The listing builds one solid part. Answer for the finished solid, in the listing's coordinates (mm). Face numbers are marked on the shaded views. Coordinates: 2 decimals unless noted, no trailing zeros. Order: outer loops, then holes, each group sorted by start corner. A loop starts at its lowest first (then second) coordinate and runs counter-clockwise, first axis right, second up.
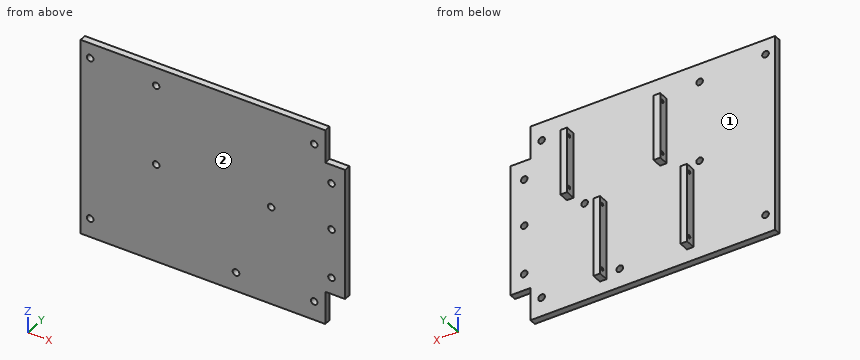
from build123d import *

# Parameters (mm, degrees)
SKETCH1_W               = 508
SKETCH1_H               = 381
BOSS_EXTRUDE1_DEPTH     = 12.7
SKETCH5_W               = 12.7
SKETCH5_H               = 127
BOSS_EXTRUDE2_DEPTH     = 19.05
SKETCH6_W               = 12.7
SKETCH6_H               = 127
BOSS_EXTRUDE3_DEPTH     = 19.05
SKETCH7_W               = 12.7
SKETCH7_H               = 152.4
BOSS_EXTRUDE6_DEPTH     = 19.05
CUT_EXTRUDE1_DEPTH      = 445.227773783
CUT_EXTRUDE1_DEPTH_BACK = 445.227773783
SKETCH8_R               = 3.175
CUT_EXTRUDE2_DEPTH      = 389.026049383
CUT_EXTRUDE2_DEPTH_BACK = 389.026049383
SKETCH9_R               = 3.175
SKETCH10_W              = 38.1
SKETCH10_H              = 63.5
CUT_EXTRUDE3_DEPTH      = 319.070986574
SKETCH11_W              = 38.1
SKETCH11_H              = 63.5
CUT_EXTRUDE4_DEPTH      = 319.070986574
CUT_EXTRUDE5_DEPTH      = 319.070986574
CUT_EXTRUDE5_DEPTH_BACK = 319.070986574
SKETCH13_R              = 6.35


with BuildPart() as part:
    # Sketch1 → Boss-Extrude1 (new body)
    with BuildSketch(Plane(origin=(0, 0, 0), x_dir=(1, 0, 0), z_dir=(0, 1, 0))):
        Rectangle(SKETCH1_W, SKETCH1_H)
    extrude(amount=BOSS_EXTRUDE1_DEPTH)

    # Sketch5 → Boss-Extrude2 (add)
    with BuildSketch(Plane(origin=(0, 12.7, 0), x_dir=(1, 0, 0), z_dir=(0, 1, 0))):
        with Locations((139.7, -82.55)):
            Rectangle(SKETCH5_W, SKETCH5_H)
    extrude(amount=BOSS_EXTRUDE2_DEPTH)

    # Sketch6 → Boss-Extrude3 (add)
    with BuildSketch(Plane(origin=(0, 12.7, 0), x_dir=(1, 0, 0), z_dir=(0, 1, 0))):
        with Locations((-39.37, -82.55)):
            Rectangle(SKETCH6_W, SKETCH6_H)
    extrude(amount=BOSS_EXTRUDE3_DEPTH)

    # Sketch7 → Boss-Extrude6 (add)
    with BuildSketch(Plane(origin=(0, 12.7, 0), x_dir=(1, 0, 0), z_dir=(0, 1, 0))):
        with Locations((76.2, 88.9)):
            Rectangle(SKETCH7_W, SKETCH7_H)
        with Locations((-90.932, 88.9)):
            Rectangle(SKETCH7_W, SKETCH7_H)
    extrude(amount=BOSS_EXTRUDE6_DEPTH)

    # Sketch8 → Cut-Extrude1 (cut, two sides: drawn at the far end of the back side and taken through both)
    with BuildSketch(Plane(origin=(146.05, 0, 0), x_dir=(0, 0, -1), z_dir=(1, 0, 0)).offset(-CUT_EXTRUDE1_DEPTH_BACK)):
        with Locations((-31.75, 25.4)):
            Circle(SKETCH8_R)
        with Locations((-133.35, 25.4)):
            Circle(SKETCH8_R)
    extrude(amount=CUT_EXTRUDE1_DEPTH + CUT_EXTRUDE1_DEPTH_BACK, mode=Mode.SUBTRACT)

    # Sketch9 → Cut-Extrude2 (cut, two sides: drawn at the far end of the back side and taken through both)
    with BuildSketch(Plane(origin=(82.55, 0, 0), x_dir=(0, 0, -1), z_dir=(1, 0, 0)).offset(-CUT_EXTRUDE2_DEPTH_BACK)):
        with Locations((25.4, 25.4)):
            Circle(SKETCH9_R)
        with Locations((152.4, 25.4)):
            Circle(SKETCH9_R)
    extrude(amount=CUT_EXTRUDE2_DEPTH + CUT_EXTRUDE2_DEPTH_BACK, mode=Mode.SUBTRACT)

    # Sketch10 → Cut-Extrude3 (cut, through all)
    with BuildSketch(Plane(origin=(0, 12.7, 0), x_dir=(1, 0, 0), z_dir=(0, 1, 0))):
        with Locations((234.95, -158.75)):
            Rectangle(SKETCH10_W, SKETCH10_H)
    extrude(amount=-CUT_EXTRUDE3_DEPTH, mode=Mode.SUBTRACT)

    # Sketch11 → Cut-Extrude4 (cut, through all)
    with BuildSketch(Plane(origin=(0, 12.7, 0), x_dir=(1, 0, 0), z_dir=(0, 1, 0))):
        with Locations((234.95, 158.75)):
            Rectangle(SKETCH11_W, SKETCH11_H)
    extrude(amount=-CUT_EXTRUDE4_DEPTH, mode=Mode.SUBTRACT)

    # Sketch13 → Cut-Extrude5 (cut, two sides: drawn at the far end of the back side and taken through both)
    with BuildSketch(Plane(origin=(0, 12.7, 0), x_dir=(1, 0, 0), z_dir=(0, 1, 0)).offset(-CUT_EXTRUDE5_DEPTH_BACK)):
        with Locations(Location((227.907081751, 0, 0), (0, 0, 270))):
            Circle(SKETCH13_R)
        with Locations(Location((111.925251719, 0, 0), (0, 0, 270))):
            Circle(SKETCH13_R)
        with Locations(Location((-108.969473195, 0, 0), (0, 0, 270))):
            Circle(SKETCH13_R)
        with Locations(Location((227.907081751, -90.673413336, 0), (0, 0, 270))):
            Circle(SKETCH13_R)
        with Locations(Location((227.907081751, 94.901161445, 0), (0, 0, 270))):
            Circle(SKETCH13_R)
        with Locations(Location((194.548146226, 154.151481102, 0), (0, 0, 270))):
            Circle(SKETCH13_R)
        with Locations(Location((194.548146226, -155.144429721, 0), (0, 0, 270))):
            Circle(SKETCH13_R)
        with Locations(Location((-235.634199607, -161.494429721, 0), (0, 0, 270))):
            Circle(SKETCH13_R)
        with Locations(Location((-235.634199607, 154.151481102, 0), (0, 0, 270))):
            Circle(SKETCH13_R)
        with Locations(Location((44.45, 154.151481102, 0), (0, 0, 270))):
            Circle(SKETCH13_R)
        with Locations(Location((-108.969473196, -155.144429721, 0), (0, 0, 270))):
            Circle(SKETCH13_R)
    extrude(amount=CUT_EXTRUDE5_DEPTH + CUT_EXTRUDE5_DEPTH_BACK, mode=Mode.SUBTRACT)


solid = part.part
1) Section B-B (z = 57) is taken. Give the vertices of the cut face in (x, y), then the cut area to 3 significant figures.
2) Section A-A (x = 44.45) is taken. Give the vertices of the cut face in (y, z).
3) Consider L1, parallel to Z at x = -91.75, y = 25.4 (3 decimals); L2, parallel to Z at x = 194.5, y = 9; L3, parallel to X at y = 26.5, z = -73. Determine where each line is inside the solid, lowest interval first.
4) Section D-D (y = 7.5) is taken. Give the number of separate pieces and of enclosed holes in the cut face, then the cut area to 3 significant figures.
5) Determine the mould class of the marked faces 1 and 2 for opening direction X: released by +X, released by -X, zero draft, split by the parting line, or undercut.
6) Each of these flat-tipped pins is pushed along its axis until it touches: P1, Ø20.5, axis at x = 111.93, z = 0, coming from the +Y side; P2, Ø10, axis at y = 25.4, z = 31.75, coming from the -X side; P3, Ø2, axis at x = -85.5, y = 14.5, coming from the -Z side. Where does it stop, or does it pass through?
7) Section C-C (z = 0) is taken. Give the vertices of the cut face in (x, y).
Filled sheet:
1. outline: (-254, 0) - (254, 0) - (254, 12.7) - (146.05, 12.7) - (146.05, 31.75) - (133.35, 31.75) - (133.35, 12.7) - (-33.02, 12.7) - (-33.02, 31.75) - (-45.72, 31.75) - (-45.72, 12.7) - (-254, 12.7) - close
1. area: 6,940 mm2
2. outline: (0, -190.5) - (12.7, -190.5) - (12.7, -160.5) - (0, -160.5) - close; (0, -147.8) - (12.7, -147.8) - (12.7, 190.5) - (0, 190.5) - close
3. L1: z = -165.1 to -155.575, -149.225 to -28.575, -22.225 to -12.7
3. L2: z = -190.5 to -160.5, -147.8 to 148.79, 161.49 to 190.5
3. L3: x = -97.28 to -84.58, 69.85 to 82.55
4. separate pieces: 1
4. enclosed holes: 11
4. area: 187,000 mm2
5. face 1: undercut
5. face 2: zero draft
6. P1: stops at y = 12.7
6. P2: stops at x = -45.72
6. P3: stops at z = -165.1
7. outline: (-254, 0) - (-115.32, 0) - (-115.32, 12.7) - (-254, 12.7) - close; (-102.62, 0) - (105.58, 0) - (105.58, 12.7) - (-102.62, 12.7) - close; (118.28, 0) - (221.56, 0) - (221.56, 12.7) - (118.28, 12.7) - close; (234.26, 0) - (254, 0) - (254, 12.7) - (234.26, 12.7) - close
